```python
from build123d import *

# Parameters (mm, degrees)
BOSS_EXTRUDE1_DEPTH      = 0.6
BOSS_EXTRUDE1_DEPTH_BACK = 0.6
SKETCH1_W                = 11.8
SKETCH1_H                = 17.5
BOSS_EXTRUDE2_DEPTH      = 2
BOSS_EXTRUDE2_DEPTH_BACK = 2
SKETCH1_3_W              = 7.8
SKETCH1_3_H              = 14.5
SKETCH1_3_W_2            = 5.8
SKETCH1_3_H_2            = 12.5
CUT_EXTRUDE1_DEPTH       = 11.741159155
CUT_EXTRUDE1_DEPTH_BACK  = 11.741159155
SKETCH1_4_W              = 5.8
SKETCH1_4_H              = 12.5
FILLET1_R                = 1


with BuildPart() as part:
    # Sketch1 → Boss-Extrude1 (new, two sides: drawn at the far end of the back side and taken through both)
    with BuildSketch(Plane.XY.offset(-BOSS_EXTRUDE1_DEPTH_BACK)):
        Rectangle(SKETCH1_W, SKETCH1_H)
    extrude(amount=BOSS_EXTRUDE1_DEPTH + BOSS_EXTRUDE1_DEPTH_BACK)

    # Sketch1<3> → Boss-Extrude2 (add, two sides: drawn at the far end of the back side and taken through both)
    with BuildSketch(Plane.XY.offset(-BOSS_EXTRUDE2_DEPTH_BACK)):
        Rectangle(SKETCH1_3_W, SKETCH1_3_H)
        Rectangle(SKETCH1_3_W_2, SKETCH1_3_H_2, mode=Mode.SUBTRACT)
    extrude(amount=BOSS_EXTRUDE2_DEPTH + BOSS_EXTRUDE2_DEPTH_BACK)

    # Sketch1<4> → Cut-Extrude1 (cut, two sides: drawn at the far end of the back side and taken through both)
    with BuildSketch(Plane.XY.offset(-CUT_EXTRUDE1_DEPTH_BACK)):
        Rectangle(SKETCH1_4_W, SKETCH1_4_H)
    extrude(amount=CUT_EXTRUDE1_DEPTH + CUT_EXTRUDE1_DEPTH_BACK, mode=Mode.SUBTRACT)

    # Fillet1
    fillet1_edges = [part.edges().sort_by_distance(p)[0] for p in [
        (-3.9, -7.25, -1.3),
        (-3.9, 7.25, -1.3),
        (3.9, 7.25, -1.3),
        (3.9, -7.25, -1.3),
        (-3.9, -7.25, 1.3),
        (-3.9, 7.25, 1.3),
        (3.9, 7.25, 1.3),
        (3.9, -7.25, 1.3),
        (-5.9, 8.75, 0),
        (5.9, 8.75, 0),
        (5.9, -8.75, 0),
        (-5.9, -8.75, 0),
    ]]
    fillet(fillet1_edges, radius=FILLET1_R)


solid = part.part
```
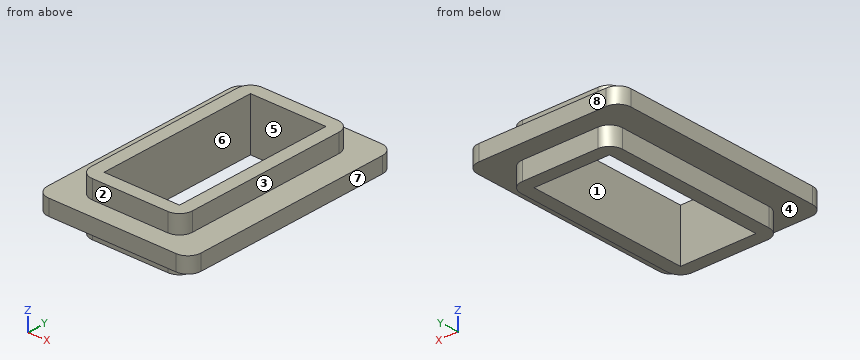
Work out the finished part from the listing and answer in its coordinate system (mm). Face numbers are marked on the shaded views. A direction names the side the tool comes from. Give positions to 0.01 mm unless a question says otherwise; leave off trailing zeros. Write each loop counter-clockwise with the first axis right and the second up, starting at its lowest first coordinate (ties: lowest second). Pieces come first, ordered by that corner, then holes. Notation, with made-up numbers: (33.25, 8.5) -> (67.25, 8.5) arc R28 cw to (67.25, 28.5) -> close; hole circle Ø11 at (-27, 11.25). An arc over 180 degrees is marked (long way). Write item = value, one per line.
Q1. Flat-ended cylindrical pins translate along their axes: pin 1 Ø0.7 at (y, z) = (0.5, 1) entering from +X; pin 2 Ø1.5 at (x, z) = (-1.5, -1.5) entering from -Y; pin 3 Ø1.5 at (x, z) = (-4, -1.5) entering from +Y. Find the tip coordinate at first contact, or state that the pin passes through.
Computed values:
pin_1 = 3.9
pin_2 = -7.25
pin_3 = 7.19
Q2. Section A-A on y = -2.5 is taken. Determine the outline of the cut face in (x, z), and give its area (3 significant figures).
Computed values:
outline = (-5.9, -0.6) -> (-3.9, -0.6) -> (-3.9, -2) -> (-2.9, -2) -> (-2.9, 2) -> (-3.9, 2) -> (-3.9, 0.6) -> (-5.9, 0.6) -> close; (2.9, -2) -> (3.9, -2) -> (3.9, -0.6) -> (5.9, -0.6) -> (5.9, 0.6) -> (3.9, 0.6) -> (3.9, 2) -> (2.9, 2) -> close
area = 12.8 mm^2
Q3. Section B-B on x = -1.5 is taken. Determine the outline of the cut face in (y, z).
Computed values:
outline = (-8.75, -0.6) -> (-7.25, -0.6) -> (-7.25, -2) -> (-6.25, -2) -> (-6.25, 2) -> (-7.25, 2) -> (-7.25, 0.6) -> (-8.75, 0.6) -> close; (6.25, -2) -> (7.25, -2) -> (7.25, -0.6) -> (8.75, -0.6) -> (8.75, 0.6) -> (7.25, 0.6) -> (7.25, 2) -> (6.25, 2) -> close
Q4. Section D-D on x = -3.25 is taken. Determine the outline of the cut face in (y, z).
Computed values:
outline = (-8.75, -0.6) -> (-7.19, -0.6) -> (-7.19, -2) -> (7.19, -2) -> (7.19, -0.6) -> (8.75, -0.6) -> (8.75, 0.6) -> (7.19, 0.6) -> (7.19, 2) -> (-7.19, 2) -> (-7.19, 0.6) -> (-8.75, 0.6) -> close
Q5. For a pull along X with two mould halves and no side action, classify the marked faces 5, 6, 7 and 8 as pulls with the +X half, pulls with the -X half, needs draft (parallel to the pull), parting line crosses it, or undercut.
Computed values:
face_5 = undercut
face_6 = undercut
face_7 = pulls with the +X half
face_8 = needs draft
Q6. Consider line 1 along X through (y, z) = (4, -1.55); line 2 along X through (y, z) = (2.5, -0.1); line 3 along Y through (x, z) = (2, -1.55). Determine where each line is inside the solid, lowest interval first.
Computed values:
line_1 = -3.9 to -2.9, 2.9 to 3.9
line_2 = -5.9 to -2.9, 2.9 to 5.9
line_3 = -7.25 to -6.25, 6.25 to 7.25
Q7. Section C-C on z = -0.4 is taken. Determine the outline of the cut face in (x, y).
Computed values:
outline = (-5.9, -7.75) arc R1 ccw to (-4.9, -8.75) -> (4.9, -8.75) arc R1 ccw to (5.9, -7.75) -> (5.9, 7.75) arc R1 ccw to (4.9, 8.75) -> (-4.9, 8.75) arc R1 ccw to (-5.9, 7.75) -> close; hole (-2.9, -6.25) -> (2.9, -6.25) -> (2.9, 6.25) -> (-2.9, 6.25) -> close
Q8. A tool of negligible diameter and unlimited length cuts with its end or side. For the marked faces 1, 2, 3 and 4, from which of +Z, -Z, +X, -X, +Y, -Y can it reach the whole face along a straight path? Write none if from no direction.
Computed values:
face_1 = +Z, -Z
face_2 = +Z, +X, -X, -Y
face_3 = +Z, +X, +Y, -Y
face_4 = -Z
